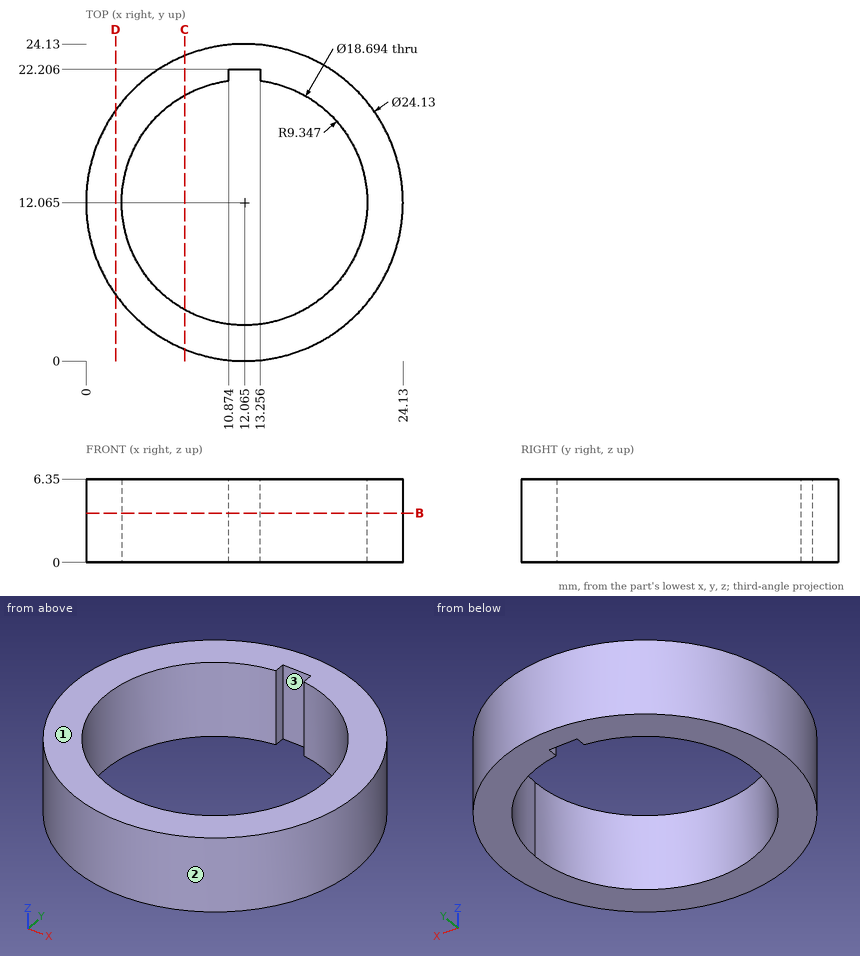
Drawing for the job (mm, zero at the part's lowest x, y, z). Round coordinates to 2 decimals unless told otherwise and drop trailing zeros. Loops run counter-clockwise (first coordinate to the right, second up) from the corner with the lowest first, then second, coordinate; pieces in that order, holes last. Notation, with made-up numbers: (-10.75, 19.25) -> (15.25, 19.25) arc R16 ccw to (15.25, 40.25) -> close; hole circle Ø8 at (40, 35.25). An arc over 180 degrees is marked (long way). Answer in a Markdown table with one row per item.
Item 1: Drill centre lines: L1, parallel to X at y = 9.25, z = 2.5; L2, parallel to X at y = 17.5, z = 6 (1 decimal); L3, parallel to Y at x = 10.75, z = 6. Where is each one in solid material? Low to high. Write a range as [from, to].
Answers below:
| item | result |
|---|---|
| L1 | x = [0.33, 3.15], [20.98, 23.8] |
| L2 | x = [1.3, 4.5], [19.7, 22.8] |
| L3 | y = [0.07, 2.81], [21.32, 24.06] |
Item 2: Saw through at B-B (z = 3.75). Write the cut outline in (x, y) (1 decimal).
Answers below:
| item | result |
|---|---|
| outline | circle Ø24.1 at (12.1, 12.1); hole (10.9, 21.3) arc R9.3 ccw (long way) to (13.3, 21.3) -> (13.3, 22.2) -> (10.9, 22.2) -> close |
Item 3: Saw through at D-D (x = 2.25). Write the cut outline in (y, z).
Answers below:
| item | result |
|---|---|
| outline | (5.05, 0) -> (19.08, 0) -> (19.08, 6.35) -> (5.05, 6.35) -> close |
Item 4: Mould opens along Y. For the marked faces 1, 2 and 3 say: +Y half, -Y half, draft (parallel to the pull), parting line (faces both ways), or undercut.
Answers below:
| item | result |
|---|---|
| face 1 | draft |
| face 2 | parting line |
| face 3 | undercut |
Item 5: Saw through at C-C (x = 7.5). Write the cut outline in (y, z).
Answers below:
| item | result |
|---|---|
| outline | (0.9, 0) -> (3.91, 0) -> (3.91, 6.35) -> (0.9, 6.35) -> close; (20.22, 0) -> (23.23, 0) -> (23.23, 6.35) -> (20.22, 6.35) -> close |
Item 6: Pin check, flat tips, straight feed: pin 1 (1 mm diameter, centred on x = 13, z = 1, fed in from +Y); pin 2 (0.7 mm diameter, centred on y = 21.5, z = 4, fed in from -X) (1 decimal); pin 3 (1 mm diameter, centred on x = 20, z = 2, fed in from -Y). Stop position of each tip, or through.
Answers below:
| item | result |
|---|---|
| pin 1 | stops at y = 24.12 |
| pin 2 | stops at x = 4.1 |
| pin 3 | stops at y = 2.56 |
